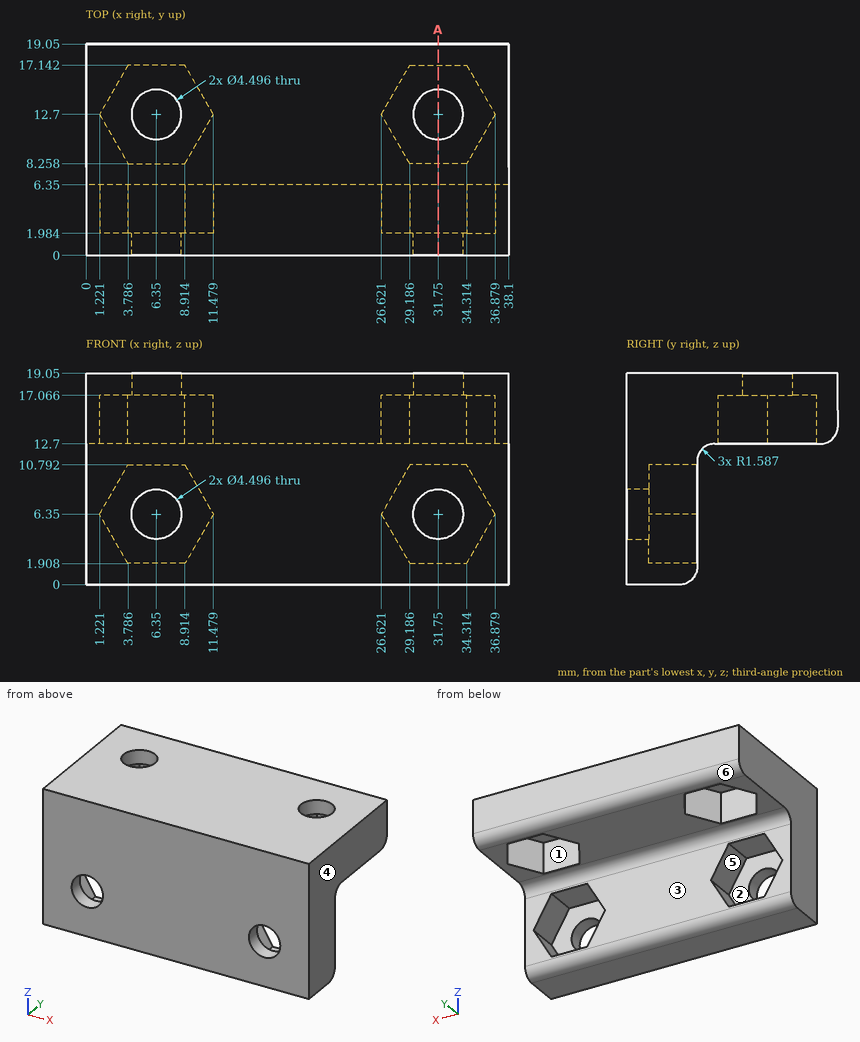
The figure shows three views and two pictorial views of one solid part (mm, origin at its lowest corner). Answer the questions. A direction names the side the tool comes from. Round coordinates to 2 decimals unless told otherwise and drop trailing zeros. Use one line per item in the form item = value. Start each with the question number.
Item 1: A cutting plane is placed at A-A (x = 31.75). Give the number of separate pieces and of enclosed holes in the cut face, plus the area to 3 significant figures.
Item 2: Find the intervals of material crossed by line 1 (X direction, y = 12.7, z = 18.6); line 2 (Z direction, x = 4, y = 3.25); line 3 (X direction, y = 4.25, z = 5.25) (1 decimal), in increasing order. Write a range as [from, to].
Item 3: Determine the mould class of the marked faces 4, 5 and 6 for opening direction Z: +Z half, -Z half, draft (parallel to the pull), parting line (faces both ways), or undercut.
Item 4: A tool of negligible diameter and unlimited length cuts with its end or side. For the marked faces 1, 2 and 3, from which of +Z, -Z, +X, -X, +Y, -Y can it reach the whole face along a straight path? Write none if from no direction.
Item 5: Flat-ended cylindrical pins translate along their axes: pin 1 Ø2 at (x, z) = (7.5, 5.5) entering from -Y; pin 2 Ø2 at (x, z) = (26, 3) entering from +Y; pin 3 Ø5 at (x, y) = (28.5, 11.5) entering from -Z; pin 4 Ø4.5 at (x, y) = (32.5, 12) entering from -Z. Find the tip coordinate at first contact, or state that the pin passes through.
The answers:
q1.separate_pieces = 3
q1.enclosed_holes = 0
q1.area = 106 mm^2
q2.line_1 = [0, 4.1], [8.6, 29.5], [34, 38.1]
q2.line_2 = [0, 1.91], [10.79, 19.05]
q2.line_3 = [0, 1.9], [10.8, 27.3], [36.2, 38.1]
q3.face_4 = draft
q3.face_5 = undercut
q3.face_6 = -Z half
q4.face_1 = -Z
q4.face_2 = +Y
q4.face_3 = -Z, +X, -X, +Y
q5.pin_1 = 0
q5.pin_2 = 6.35
q5.pin_3 = 12.7
q5.pin_4 = 17.07
